Autodesk Inventor part; units mm, degrees
ref_plane "YZ Plane" through (0, 0, 0) normal (1, 0, 0) x (0, 1, 0)
ref_plane "XZ Plane" through (0, 0, 0) normal (0, 1, 0) x (-1, 0, 0)
ref_plane "XY Plane" through (0, 0, 0) normal (0, 0, 1) x (1, 0, 0)
sketch "Esboço1" plane through (0, 0, 0) normal (0, 0, 1) x (1, 0, 0)
  line L0 (-17, 11) -> (17, 11) construction
  line L1 (17, 11) -> (17, -7) construction
  line L2 (17, -7) -> (-17, -7) construction
  line L3 (-17, -7) -> (-17, 11) construction
  line L4 (-14, 20.4248) -> (-14, -25.3484) construction
  line L5 (14, 20.4248) -> (14, -25.3484) construction
  line L6 (0, 20.9223) -> (0, -24.8509) construction
  line L7 (-26.3196, 0) -> (26.3196, 0) construction
  line L8 (-26.3196, 5) -> (26.3196, 5) construction
  line L9 (-15.5, 15.1736) -> (-15.5, -30.5996) construction
  line L10 (15.5, 20.4248) -> (15.5, -25.3484) construction
  line L11 (0, 0) -> (-21.4941, -25.6157) construction
  line L12 (0, 0) -> (11.7474, -14) construction
  line L13 (-8, 20.4248) -> (-8, -25.3484) construction
  line L14 (-5, 20.4248) -> (-5, -25.3484) construction
  line L15 (5, 20.9223) -> (5, -24.8509) construction
  line L16 (8, 20.9223) -> (8, -24.8509) construction
  line L17 (-26.3196, 3.5) -> (26.3196, 3.5) construction
  line L18 (-17, 11) -> (-17, 5)
  line L19 (-17, 5) -> (-15.5, 3.5)
  line L20 (-15.5, 3.5) -> (-15.5, -7)
  line L21 (17, 5) -> (17, 11)
  line L22 (26.3196, 10) -> (-26.3196, 10) construction
  line L23 (-17, 11) -> (-8, 11)
  line L24 (17, 11) -> (8, 11)
  line L25 (-8, 11) -> (-7.6714, 11) construction
  line L26 (-8, 11) -> (-7.5337, 10)
  line L27 (-8, 11) -> (-6.8966, 11) construction
  line L28 (-5, 11) -> (-3.8966, 11) construction
  line L29 (8, 11) -> (7.5337, 10)
  line L30 (15.5, -7) -> (15.5, 3.5)
  line L31 (17, 5) -> (15.5, 3.5)
  line L32 (-26.3196, -11) -> (26.3196, -11) construction
  line L33 (-7.5337, 10) -> (7.5337, 10)
  line L34 (-8, -7) -> (-5, -11)
  line L35 (8, -7) -> (5, -11)
  line L36 (-5, -11) -> (5, -11)
  line L37 (-8, -7) -> (-15.5, -7)
  line L38 (8, -7) -> (15.5, -7)
  circle A0 centre (0, 0) radius 7.5
  point P0 (0, 11)
  point P1 (0, 5)
  point P2 (0, -11)
  dimension "d0" = 34
  dimension "d1" = 18
  dimension "d2" = 14
  dimension "d3" = 14
  dimension "d4" = 11
  dimension "d5" = 6
  dimension "d6" = 1.5
  dimension "d7" = 1.5
  dimension "d8" = 40
  dimension "d9" = 40
  dimension "d10" = 5
  dimension "d11" = 5
  dimension "d12" = 8
  dimension "d13" = 8
  dimension "d14" = 1.5
  dimension "d15" = 1
  dimension "d18" = 115
  dimension "d20" = 115
  dimension "d21" = 22
  dimension "d22" = 15
extrude "Extrusão1" add sketch "Esboço1" along normal blind 30
sketch "Esboço2" plane through (-17, 11, 0) normal (0, 1, 0) x (1, 0, 0)
  line L0 (0, 0) -> (0, -30) construction
  line L1 (0, -15) -> (34, -15) construction
  line L2 (34, 0) -> (34, -30) construction
  line L3 (17, 0) -> (17, -29.9375) construction
  circle A0 centre (5, -24) radius 1 construction
  circle A1 centre (5, -6) radius 1 construction
  circle A2 centre (29, -6) radius 1 construction
  circle A3 centre (29, -24) radius 1 construction
  dimension "d25" = 2
  dimension "d26" = 2
  dimension "d27" = 2
  dimension "d28" = 2
  dimension "d29" = 9
  dimension "d30" = 9
  dimension "d31" = 9
  dimension "d32" = 9
  dimension "d33" = 12
  dimension "d34" = 12
  dimension "d35" = 12
  dimension "d36" = 12
hole "Furo1" at (-12, 11, 24) at (12, 11, 24) at (12, 11, 6) at (-12, 11, 6) direction (0, -1, 0) diameter 3.242 end through all
chamfer "Chanfro1" distance 1 angle 45 4 edges at (-17, 11, 15) (17, 11, 15) (15.5, -7, 15) (-15.5, -7, 15)
equation "\"d3\" = d2"
equation "\"d7\" = d6"
equation "\"d9\" = d8"
equation "\"d11\" = d10"
equation "\"d13\" = d12"
equation "\"d26\" = d25"
equation "\"d27\" = d25"
equation "\"d28\" = d25"
equation "\"d30\" = d29"
equation "\"d31\" = d29"
equation "\"d32\" = d29"
equation "\"d34\" = d33"
equation "\"d35\" = d33"
equation "\"d36\" = d33"
properties part number "PilowBlockFechadoSCS8UU"
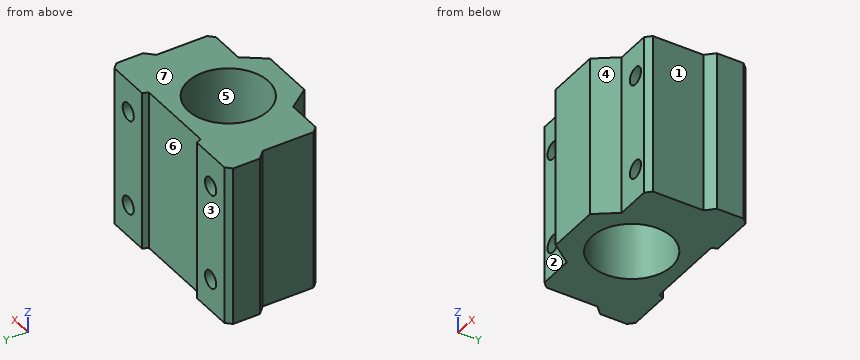
The listing builds one solid part. Answer for the finished solid, in the listing's coordinates (mm). Face numbers are marked on the shaded views. A direction names the side the tool comes from. Round coordinates to 2 decimals unless told otherwise and drop trailing zeros. Order: outer loops, then holes, each group sorted by start corner. A loop starts at its lowest first (then second) coordinate and runs counter-clockwise, first axis right, second up. Notation, with made-up numbers: (54, -16) - (73, -16) arc R16 ccw to (73, 0) - close; hole circle Ø4 at (-37, 10.25). An arc over 180 degrees is marked (long way). Put each result on its own line as item: value. Start each with the question number.
(1) Find section A-A (z = 24). State how many separate pieces and enclosed holes the cut face has, plus the area to 3 significant figures.
(2) Find section B-B (y = -4.5). Give the vertices of the cut face in (x, z), plus the area to 3 significant figures.
(3) Straight lines are drawn through the part: probe 1 along Z at (x, y) = (12, 3.5); probe 2 along X at (y, z) = (1.5, 6); probe 3 along Z at (x, y) = (-11, 5.5). For each, find the intervals that lie inside material, in ascending order. Write a range as from..to.
(4) Find section C-C (x = 0). Give the vertices of the cut face in (y, z), plus the area to 3 significant figures.
(5) Given P1, Ø12, axis at x = 0, z = 10, coming from the +Y side; P2, Ø1, axis at y = 0.5, z = 21, coming from the +X side; P3, Ø2, axis at x = 12.5, z = 17.5, coming from the -Y side, each flat-ended and moving along its own axis, determine where each tip first touches the part or whether it passes through.
(6) Determine the mould class of the marked faces 4, 5, 6 and 7 for opening direction X: released by +X, released by -X, zero draft, split by the parting line, or undercut.
(7) Find section D-D (z = 11). Give the vertices of the cut face in (x, y).
(8) For the marked faces 1, 2 and 3, determine the directions among +Z, -Z, +X, -X, +Y, -Y from which every point of the face is accessible in a straight line to the end or side of a thin tool.
Reply:
1. separate pieces: 3
1. enclosed holes: 1
1. area: 319 mm^2
2. outline: (-15.5, 0) - (-6, 0) - (-6, 30) - (-15.5, 30) - close; (6, 0) - (15.5, 0) - (15.5, 30) - (6, 30) - close; hole circle Ø3.24 at (-12, 6); hole circle Ø3.24 at (-12, 24); hole circle Ø3.24 at (12, 6); hole circle Ø3.24 at (12, 24)
2. area: 537 mm^2
3. probe 1: 0..4.38, 7.62..22.38, 25.62..30
3. probe 2: -15.5..-13.62, -10.38..-7.35, 7.35..10.38, 13.62..15.5
3. probe 3: 0..4.72, 7.28..22.72, 25.28..30
4. outline: (-11, 0) - (-7.5, 0) - (-7.5, 30) - (-11, 30) - close; (7.5, 0) - (10, 0) - (10, 30) - (7.5, 30) - close
4. area: 180 mm^2
5. P1: y = 10
5. P2: x = 15.5
5. P3: y = -7
6. face 4: released by +X
6. face 5: undercut
6. face 6: undercut
6. face 7: zero draft
7. outline: (-17, 5) - (-15.5, 3.5) - (-15.5, -6) - (-14.5, -7) - (-8, -7) - (-5, -11) - (5, -11) - (8, -7) - (14.5, -7) - (15.5, -6) - (15.5, 3.5) - (17, 5) - (17, 10) - (16, 11) - (8, 11) - (7.53, 10) - (-7.53, 10) - (-8, 11) - (-16, 11) - (-17, 10) - close; hole circle Ø15 at (0, 0)
8. face 1: +Z, -Z, +X, -Y
8. face 2: +Z, -Z, -X, -Y
8. face 3: +Z, -Z, +X, -X, +Y
